```python
from build123d import *

# Parameters (mm, degrees)
SKETCH054_W             = 6.6
SKETCH054_H             = 12
PAD012_DEPTH            = 2
SKETCH055_W             = 6.6
SKETCH055_H             = 5
PAD013_DEPTH            = 0.8
SKETCH056_R             = 1.8
POCKET014_DEPTH         = 2
BODY005_PLACEMENT_ANGLE = 180


with BuildPart() as part:
    # Sketch054 → Pad012 (new body)
    with BuildSketch(Plane.XY):
        with Locations((3.3, 6)):
            Rectangle(SKETCH054_W, SKETCH054_H)
    extrude(amount=PAD012_DEPTH)

    # Sketch055 (on Face6 of Pad012) → Pad013 (join)
    with BuildSketch(Plane.XY.offset(2)):
        with Locations((3.3, 9.5)):
            Rectangle(SKETCH055_W, SKETCH055_H)
    extrude(amount=PAD013_DEPTH)

    # Sketch056 (on Face7 of Pad013) → Pocket014 (cut)
    with BuildSketch(Plane.XY.offset(2)):
        with Locations((3, 3.4)):
            Circle(SKETCH056_R)
    extrude(amount=-POCKET014_DEPTH, mode=Mode.SUBTRACT)


with BuildPart() as part_1:
    # Body005 placement: moved
    add(part.part.moved(Location((-17, 72.5, 8))).rotate(Axis((-17, 72.5, 8), (1, 0, 0)), BODY005_PLACEMENT_ANGLE))


solid = part_1.part
```
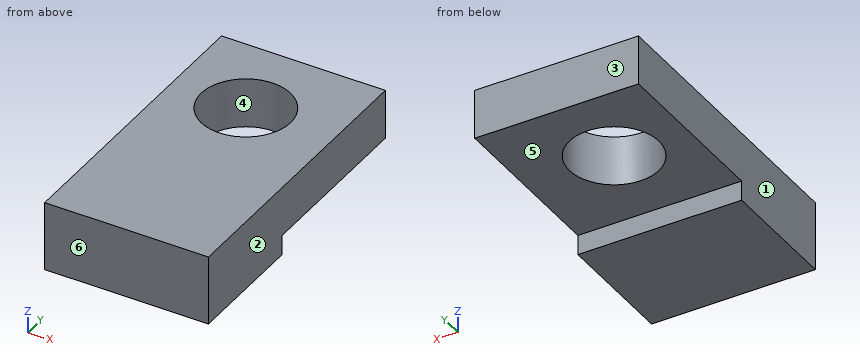
Input: part model. Units: mm. Frame: model coordinates. Face numbers are marked on the shaded views. A direction names the side the tool comes from. Coordinates: 2 decimals unless noted, no trailing zeros. Order: outer loops, then holes, each group sorted by start corner. A loop starts at its lowest first (then second) coordinate and runs counter-clockwise, first axis right, second up. Notation, with made-up numbers: (88.25, 78) - (92.25, 78) arc R18 ccw to (92.25, 94) - close; hole circle Ø1 at (53, -6.5). An arc over 180 degrees is marked (long way). Put each result on its own line as item: value.
1. Cut plane C-C on z = 6.7. Return the cut outline in (x, y), then the cut area to 3 significant figures.
Report:
outline: (-17, 60.5) - (-10.4, 60.5) - (-10.4, 72.5) - (-17, 72.5) - close; hole circle Ø3.6 at (-14, 69.1)
area: 69.0 mm2
2. Reachability of the marked faces 5 and 6 from +Z, -Z, +X, -X, +Y, -Y: full face, straight path, thin tool, end or side. Return the list, or none.
Report:
face 5: -Z, +X, -X, +Y
face 6: +Z, -Z, +X, -X, -Y
3. Contact query for a flat-ended pin moving along its axis: pin 1 Ø1 at (x, y) = (-14.5, 67.5) entering from -Z. Output: stop coordinate, or through.
Report:
pin 1: stops at z = 6
4. Cut plane B-B on x = -14. Return the cut outline in (y, z).
Report:
outline: (60.5, 5.2) - (65.5, 5.2) - (65.5, 6) - (67.3, 6) - (67.3, 8) - (60.5, 8) - close; (70.9, 6) - (72.5, 6) - (72.5, 8) - (70.9, 8) - close
5. Draft query along X for the marked faces 1, 2, 3 and 4. Return one class per face: pulls with the +X half, pulls with the -X half, needs draft (parallel to the pull), parting line crosses it, or undercut.
Report:
face 1: pulls with the -X half
face 2: pulls with the +X half
face 3: needs draft
face 4: undercut
6. Cut plane A-A on y = 69.1. Return the cut outline in (x, z).
Report:
outline: (-17, 6) - (-15.8, 6) - (-15.8, 8) - (-17, 8) - close; (-12.2, 6) - (-10.4, 6) - (-10.4, 8) - (-12.2, 8) - close
7. Cut plane D-D on x = -11.5. Return the cut outline in (y, z), then the cut area to 3 significant figures.
Report:
outline: (60.5, 5.2) - (65.5, 5.2) - (65.5, 6) - (72.5, 6) - (72.5, 8) - (60.5, 8) - close
area: 28.0 mm2
8. Line query: line 1 along Y through (x, z) = (-14, 7.3); line 2 along X through (y, z) = (69.1, 6.85); line 3 along Z through (x, y) = (-16.5, 70.25). Output: solid intervals per line, ascending.
Report:
line 1: y = 60.5 to 67.3, 70.9 to 72.5
line 2: x = -17 to -15.8, -12.2 to -10.4
line 3: z = 6 to 8
